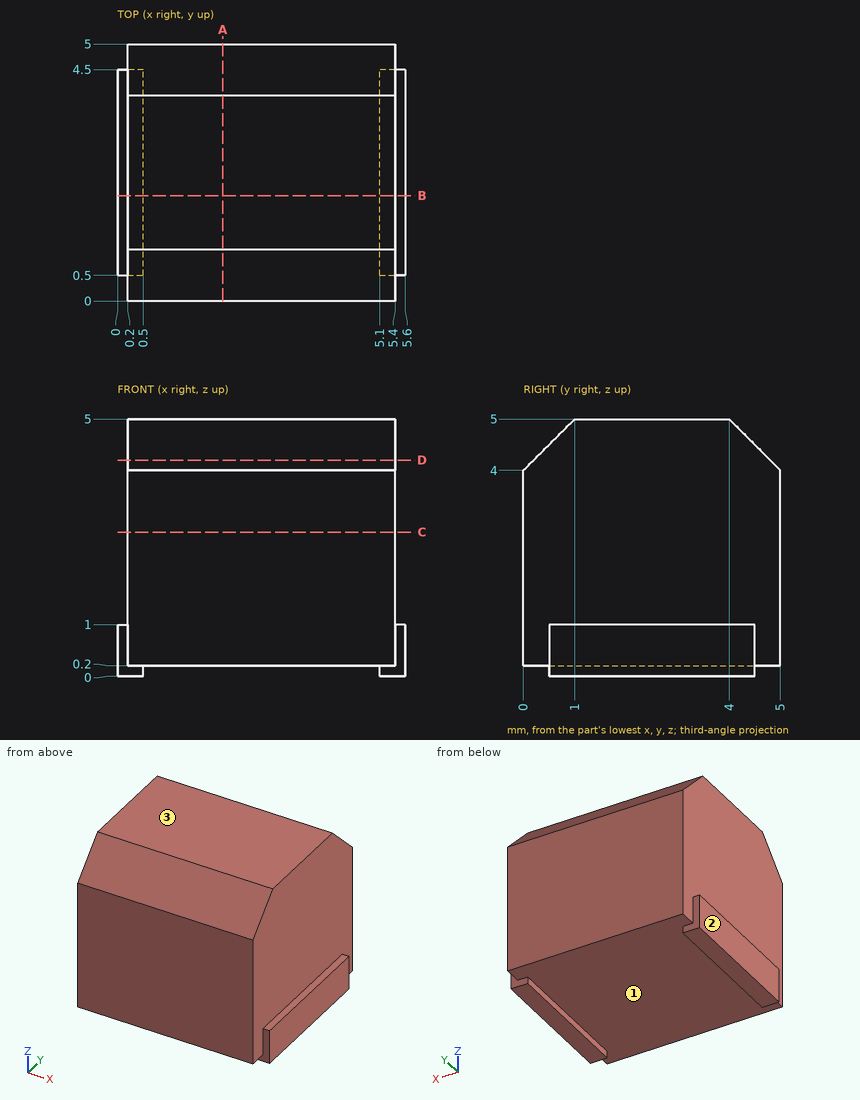
Input: dimensioned drawing with shaded views. Units: mm. Origin: part minimum x, y, z. Round coordinates to 2 decimals unless told otherwise and drop trailing zeros. Order: outer loops, then holes, each group sorted by start corner. A loop starts at its lowest first (then second) coordinate and runs counter-clockwise, first axis right, second up. Notation, with made-up numbers: (-10, -15) - (42, -15) arc R10 cw to (42, -1) - close; hole circle Ø10 at (-14.5, -38.75). An arc over 180 degrees is marked (long way). Answer as a JSON object with one key per item and string values. Group by question number.
(1) Material intervals for probe 1 along Z at (x, y) = (4, 3.65); probe 2 along X at (y, z) = (4.15, 2.6); probe 3 along Y at (x, z) = (0.5, 4.5), sorted ascending. Write a range as from..to.
(2) Cut plane A-A (x = 2.05). Return loops of the section in (y, z), then the cut area to 3 significant figures.
(3) Cut plane B-B (y = 2.05). Return loops of the section in (x, z), then the cut area to 3 significant figures.
(4) Draft query along X for the marked faces 1, 2 and 3. Return one class per face: released by +X, released by -X, zero draft, split by the parting line, or undercut.
(5) Cut plane C-C (z = 2.8). Return loops of the section in (x, y), then the cut area to 3 significant figures.
(6) Pin query (flat end, axial travel): P1, Ø2.5, axis at x = 3.5, y = 2.5, coming from the -Z side; P2, Ø1, axis at y = 1.5, z = 3, coming from the +X side. Return the tip coordinate at first contact, or that it passes through.
(7) Cut plane D-D (z = 4.2). Return loops of the section in (x, y), then the cut area to 3 significant figures.
Here are the results:
{
 "1": {"probe 1": "z = 0.2..5", "probe 2": "x = 0.2..5.4", "probe 3": "y = 0.5..4.5"},
 "2": {"outline": "(0, 0.2) - (5, 0.2) - (5, 4) - (4, 5) - (1, 5) - (0, 4) - close", "area": "23.0 mm^2"},
 "3": {"outline": "(0, 0) - (0.5, 0) - (0.5, 0.2) - (5.1, 0.2) - (5.1, 0) - (5.6, 0) - (5.6, 1) - (5.4, 1) - (5.4, 5) - (0.2, 5) - (0.2, 1) - (0, 1) - close", "area": "25.5 mm^2"},
 "4": {"face 1": "undercut", "face 2": "released by -X", "face 3": "zero draft"},
 "5": {"outline": "(0.2, 0) - (5.4, 0) - (5.4, 5) - (0.2, 5) - close", "area": "26.0 mm^2"},
 "6": {"P1": "stops at z = 0.2", "P2": "stops at x = 5.4"},
 "7": {"outline": "(0.2, 0.2) - (5.4, 0.2) - (5.4, 4.8) - (0.2, 4.8) - close", "area": "23.9 mm^2"}
}
